Part model, mm, in its own coordinate system. Face numbers are marked on the shaded views. A direction names the side the tool comes from. Coordinates: 2 decimals unless noted, no trailing zeros. Loops run counter-clockwise (first coordinate to the right, second up) from the corner with the lowest first, then second, coordinate; pieces in that order, holes last. Notation, with made-up numbers: (72, 5) -> (86, 5) arc R24 ccw to (86, 17) -> close; hole circle Ø11 at (-25.5, 38.5). An arc over 180 degrees is marked (long way). One line per item, written item: value. Start each with the question number.
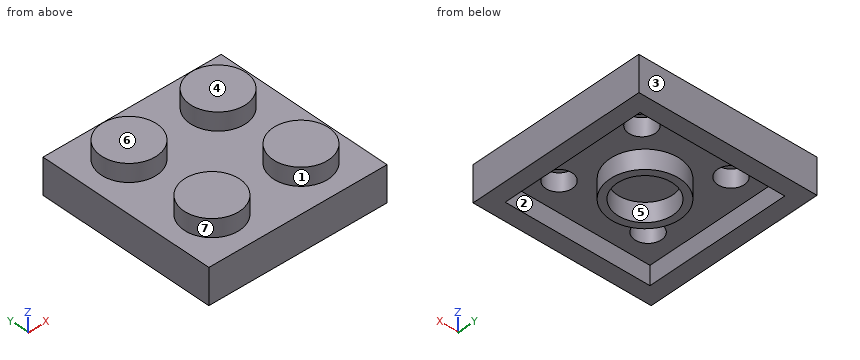
Autodesk Inventor part; units mm, degrees
ref_plane "YZ Plane" through (0, 0, 0) normal (1, 0, 0) x (0, 1, 0)
ref_plane "XZ Plane" through (0, 0, 0) normal (0, 1, 0) x (-1, 0, 0)
ref_plane "XY Plane" through (0, 0, 0) normal (0, 0, 1) x (1, 0, 0)
sketch "Sketch1" plane through (0, 0, 0) normal (0, 0, 1) x (1, 0, 0)
  line L0 (-8, 8) -> (8, 8)
  line L1 (8, 8) -> (8, -8)
  line L2 (8, -8) -> (-8, -8)
  line L3 (-8, -8) -> (-8, 8)
  point P0 (0, 0)
  dimension "d0" = 16
  dimension "d1" = 16
  dimension "d2" = 8
  dimension "d3" = 8
extrude "Extrusion1" add sketch "Sketch1" along normal blind 3.2
shell "Shell1" thickness 1.5 removed faces 1 at (-2.6667, -2.6667, 0)
sketch "Sketch2" plane through (0, 0, 3.2) normal (0, 0, 1) x (1, 0, 0)
  circle A0 centre (4, -4) radius 2.5
  line L0 (8, 8) -> (8, -8)
  line L1 (8, -8) -> (-8, -8)
  dimension "d7" = 5
  dimension "d10" = 4
  dimension "d11" = 4
extrude "Extrusion2" add sketch "Sketch2" along normal blind 1.6
sketch "Sketch3" plane through (6.5, -6.5, 1.7) normal (0, 0, -1) x (-1, 0, 0)
  circle A0 centre (2.5, 2.5) radius 2.5
  circle A1 centre (2.5, 2.5) radius 1.2
  point P0 (6.5, 6.5)
  dimension "d18" = 2.4
extrude "Extrusion3" cut sketch "Sketch3" against normal blind 1.6 contours A1
pattern_linear "Rectangular Pattern1" count 2 spacing 8 along (0, 1, 0) count 2 spacing 8 along (-1, 0, 0) of "Extrusion2", "Extrusion3"
sketch "Sketch4" plane through (6.5, -6.5, 1.7) normal (0, 0, -1) x (-1, 0, 0)
  circle A0 centre (2.5, 10.5) radius 1.2
  circle A1 centre (2.5, 2.5) radius 1.2
  line L0 (0, 13) -> (0, 0)
  line L1 (0, 0) -> (13, 0)
  circle A2 centre (6.5, 6.5) radius 3.15
  circle A3 centre (6.5, 6.5) radius 2.5
  point P0 (6.5, 6.5)
  dimension "d21" = 6.5
  dimension "d22" = 6.5
  dimension "d23" = 10.5
  dimension "d24" = 2.5
  dimension "d25" = 5
  dimension "d26" = 6.3
extrude "Extrusion4" add sketch "Sketch4" along normal up to surface (1.7 mm away) contours A2
pattern_of_one "Rectangular Pattern2"
equation "\"d0\" = 0.8 * WIDTH"
equation "\"d1\" = 0.8 * LENGTH"
equation "\"d4\" = HEIGHT"
equation "\"d21\" = 0.5 * d23 + 0.5 * d24"
equation "\"d22\" = d21"
equation "\"WIDTH\" = 2"
equation "\"HEIGHT\" = 3.2"
properties part number "3022" material "Steel"
1) Probe line 1 (Y direction, x = 4, z = 3); line 2 (X direction, y = -1, z = 0.55); line 3 (Y direction, x = 0, z = 0.7). List the from-to ranges inside material, lowest first. Write a range as from..to.
2) Pin check, flat tips, straight feed: pin 1 Ø2.5 at (x, y) = (-4.5, -4.5) entering from -Z; pin 2 Ø2 at (x, y) = (-2.5, 0) entering from +Z; pin 3 Ø0.7 at (x, y) = (4.5, 4) entering from -Z. Stop position of each tip, or through.
3) Slice it at D-D (z = 3.7). Give the cut face in (x, y).
4) Tool access for the marked faces 5, 6 and 7: list every direction of +Z, -Z, +X, -X, +Y, -Y with a clear straight run to the whole face (end or side of a thin tool).
5) Slice it at B-B (x = -6). Give the cut face in (y, z), then the cut area to 3 significant figures.
6) Slice it at A-A (z = 1.3). Give the cut face in (x, y).
7) Pull direction Y, two halves, no side cores. Call the marked faces 1, 2, 3 and 4: +Y half, -Y half, draft (parallel to the pull), parting line (faces both ways), or undercut.
Check sheet entries:
1. line 1: y = -8..-5.2, -2.8..2.8, 5.2..8
1. line 2: x = -8..-6.5, -2.99..-2.29, 2.29..2.99, 6.5..8
1. line 3: y = -8..-6.5, -3.15..-2.5, 2.5..3.15, 6.5..8
2. pin 1: stops at z = 1.7
2. pin 2: stops at z = 3.2
2. pin 3: stops at z = 3.3
3. outline: circle Ø5 at (-4, -4); circle Ø5 at (-4, 4); circle Ø5 at (4, -4); circle Ø5 at (4, 4)
4. face 5: -Z
4. face 6: +Z, +X, -X, +Y, -Y
4. face 7: +Z
5. outline: (-8, 0) -> (-6.5, 0) -> (-6.5, 1.7) -> (6.5, 1.7) -> (6.5, 0) -> (8, 0) -> (8, 3.2) -> (5.5, 3.2) -> (5.5, 4.8) -> (2.5, 4.8) -> (2.5, 3.2) -> (-2.5, 3.2) -> (-2.5, 4.8) -> (-5.5, 4.8) -> (-5.5, 3.2) -> (-8, 3.2) -> close
5. area: 38.7 mm^2
6. outline: (-8, -8) -> (8, -8) -> (8, 8) -> (-8, 8) -> close; circle Ø6.3 at (0, 0); hole (-6.5, -6.5) -> (6.5, -6.5) -> (6.5, 6.5) -> (-6.5, 6.5) -> close; hole circle Ø5 at (0, 0)
7. face 1: undercut
7. face 2: undercut
7. face 3: +Y half
7. face 4: draft
